```python
from build123d import *

# Parameters (mm, degrees)
F7_DEPTH = 21.2725
F8_R     = 2.413
F9_DEPTH = 20.0025
F10_R    = 2.413


# Not quite as in the source:
# - a variable given as a bare number and used for a length is read in inches; the dataset says mm whatever the document's units were


with BuildPart() as f7:
    # F6 (on Top) → F7 (new body)
    with BuildSketch(Plane.XY):
        Polygon((-100.2214143808, -23.920097865), (-92.4320810475, -23.920097865), (-92.4320810475, -49.320097865), (-91.1620810475, -49.320097865), (-91.1620810475, -23.920097865), (-91.1620810475, -16.1307645317), (-65.7620810475, -16.1307645317), (-65.7620810475, -14.8607645317), (-91.1620810475, -14.8607645317), (-93.2787477141, -14.8607645317), (-98.9514143808, -14.8607645317), (-98.9514143808, 10.5392354683), (-100.2214143808, 10.5392354683), (-100.2214143808, -14.8607645317), (-100.2214143808, -22.650097865), (-125.6214143808, -22.650097865), (-125.6214143808, -23.920097865), align=None)
    extrude(amount=F7_DEPTH)

    # F8 (on face) → F9 (cut)
    with BuildSketch(Plane(origin=(0, 0, 0), x_dir=(1, 0, 0), z_dir=(0, 0, -1))):
        with Locations((-95.6917477141, 19.3904311984)):
            Circle(F8_R)
    extrude(amount=-F9_DEPTH, mode=Mode.SUBTRACT)

    # F10
    f10_edges = [f7.edges().sort_by_distance(p)[0] for p in [
        (-98.104748, -19.390431, 20.0025),
    ]]
    fillet(f10_edges, radius=F10_R)


solid = f7.part
```
Here's how the part is built. I have some questions about the finished solid (model axes, mm). A direction names the side the tool comes from. Round coordinates to 2 decimals unless told otherwise and drop trailing zeros. Order: outer loops, then holes, each group sorted by start corner. A loop starts at its lowest first (then second) coordinate and runs counter-clockwise, first axis right, second up. Notation, with made-up numbers: M -25,71 L 8,71 A15 ccw 8,79 Z; hole C 0.5,80 d11. An arc over 180 degrees is marked long. One line per question, with ' | ' between items.
1) I want a section at C-C, the plane x = -102.5. Write out the boundary of the cut face in (y, z), then the cut area to 3 significant figures.
Working result:
outline: M -23.92,0 L -22.65,0 L -22.65,21.27 L -23.92,21.27 Z | area: 27.0 mm²
2) I want a section at A-A, the plane z = 13.25. Write out the boundary of the cut face in (x, y), then the cut area to 3 significant figures.
Working result:
outline: M -125.62,-23.92 L -92.43,-23.92 L -92.43,-49.32 L -91.16,-49.32 L -91.16,-16.13 L -65.76,-16.13 L -65.76,-14.86 L -98.95,-14.86 L -98.95,10.54 L -100.22,10.54 L -100.22,-22.65 L -125.62,-22.65 Z; hole C -95.69,-19.39 d4.83 | area: 193 mm²
3) I want a section at B-B, the plane y = -39. Write out the boundary of the cut face in (x, z).
Working result:
outline: M -92.43,0 L -91.16,0 L -91.16,21.27 L -92.43,21.27 Z
4) If we mould it in two halves opening along X, with no side actions, what happens to faces 4 (the face through (-79, -16.131, 10)), 5 (the face through (-100.221, -6, 10)), 6 (the face through (-93.39, -20.12, 8.67))? For each: +X half, -X half, draft (parallel to the pull), parting line (faces both ways), or undercut.
Working result:
face 4: draft | face 5: -X half | face 6: undercut
5) I need wall thicknesses on line 1 along X through (y, z) = (1, 16.5); line 2 along Y through (x, z) = (-117, 20); line 3 along X through (y, z) = (-37.5, 3.5). Which ranges of each line are inside material? Lowest first, please.
Working result:
line 1: -100.22 to -98.95 | line 2: -23.92 to -22.65 | line 3: -92.43 to -91.16
6) For faces 1 (the face through (-98.951, -2, 10)), 2 (the face through (-92.432, -36, 10)), 3 (the face through (-113, -22.65, 10)), which set-ups out of +Z, -Z, +X, -X, +Y, -Y let a thin tool reach every point of the face, with its end or its side?
Working result:
face 1: +Z, -Z, +X, +Y | face 2: +Z, -Z, -X, -Y | face 3: +Z, -Z, -X, +Y
7) For pin 1 Ø4 at (x, y) = (-95.69, -19.39) entering from -Z; pin 2 Ø10.5 at (x, z) = (-76.5, 9.5) entering from +Y; pin 3 Ø1 at (x, z) = (-108.5, 9) entering from -Y, each with a flat end and sliding along its axis, tell me the tip position at first contact or that it passes through.
Working result:
pin 1: z = 18.94 | pin 2: y = -14.86 | pin 3: y = -23.92
